```python
from build123d import *
from build123d.topology import SkipClean

# Parameters (mm, degrees)
SKETCH2_R               = 22.5
BOSS_EXTRUDE1_DEPTH     = 8
SKETCH3_R               = 5
BOSS_EXTRUDE2_DEPTH     = 70
SKETCH4_R               = 12
BOSS_EXTRUDE3_DEPTH     = 28
FILLET1_R               = 6
CUT_EXTRUDE1_DEPTH      = 85.240726493
CUT_EXTRUDE1_DEPTH_BACK = 85.240726493
SKETCH5_W               = 15
SKETCH5_H               = 20
SKETCH6_R               = 4
CUT_EXTRUDE2_DEPTH      = 28
SKETCH7_R               = 9
SKETCH7_R_2             = 4
BOSS_EXTRUDE5_DEPTH     = 12.5
FILLET3_R               = 1


with BuildPart() as part:
    # Sketch2 → Boss-Extrude1 (new body)
    with BuildSketch(Plane(origin=(0, 0, 0), x_dir=(1, 0, 0), z_dir=(0, 1, 0))):
        with Locations(Location((0, 0, 0), (0, 0, 270))):
            Circle(SKETCH2_R)
    extrude(amount=BOSS_EXTRUDE1_DEPTH)

    # Sketch3 → Boss-Extrude2 (add)
    with BuildSketch(Plane(origin=(0, 8, 0), x_dir=(1, 0, 0), z_dir=(0, 1, 0))):
        with Locations(Location((0, 0, 0), (0, 0, 270))):
            Circle(SKETCH3_R)
    extrude(amount=BOSS_EXTRUDE2_DEPTH)

    # Sketch4 → Boss-Extrude3 (add)
    with BuildSketch(Plane.XZ):
        with Locations(Location((0, 0, 0), (0, 0, 270))):
            Circle(SKETCH4_R)
    extrude(amount=BOSS_EXTRUDE3_DEPTH)

    # Fillet1
    fillet1_edges = [part.edges().sort_by_distance(p)[0] for p in [
        (0, -28, 12),
    ]]
    fillet(fillet1_edges, radius=FILLET1_R)

    # Sketch5 → Cut-Extrude1 (cut, two sides: drawn at the far end of the back side and taken through both)
    with BuildSketch(Plane(origin=(0, 0, 0), x_dir=(0, 0, -1), z_dir=(1, 0, 0)).offset(-CUT_EXTRUDE1_DEPTH_BACK)):
        with Locations((15, -18)):
            Rectangle(SKETCH5_W, SKETCH5_H)
        with Locations((-15, -18)):
            Rectangle(SKETCH5_W, SKETCH5_H)
    extrude(amount=CUT_EXTRUDE1_DEPTH + CUT_EXTRUDE1_DEPTH_BACK, mode=Mode.SUBTRACT)

    # Sketch6 → Cut-Extrude2 (cut)
    with BuildSketch(Plane(origin=(0, 0, -7.5), x_dir=(-1, 0, 0), z_dir=(0, 0, -1))):
        with Locations(Location((0, -18, 0), (0, 0, 90))):
            Circle(SKETCH6_R)
    extrude(amount=-CUT_EXTRUDE2_DEPTH, mode=Mode.SUBTRACT)

    # Sketch7 → Boss-Extrude5 (add, symmetric)
    with SkipClean():  # the faces are left unmerged after this step: merging them gives an invalid solid
        with BuildSketch(Plane.XY):
            with Locations(Location((0, -18, 0), (0, 0, 180))):
                Circle(SKETCH7_R)
            with Locations((0, -18)):
                Circle(SKETCH7_R_2, mode=Mode.SUBTRACT)
        extrude(amount=BOSS_EXTRUDE5_DEPTH, both=True)
    add(part.part.scale(1), mode=Mode.REPLACE)  # the faces are merged on a copy

    # Fillet3
    fillet3_edges = [part.edges().sort_by_distance(p)[0] for p in [
        (0, 0, -22.5),
    ]]
    fillet(fillet3_edges, radius=FILLET3_R)


solid = part.part
```
Read the model definition and answer for the solid it produces. Units are mm, in the model's axes. A direction names the side the tool comes from. Coordinates: 2 decimals unless noted, no trailing zeros. Loops run counter-clockwise (first coordinate to the right, second up) from the corner with the lowest first, then second, coordinate; pieces in that order, holes last.
(1) The mould has two halves that part along Y. Classify faces 4 (the face through (0, -8, -9)), 5 (the face through (1.172, -26.923, 10.035)), 6 (the face through (0, -28, 0)), 7 (the face through (-8.618, 4.451, 20.784)): released by +Y, released by -Y, zero draft, split by the parting line, or undercut.
Solution:
face 4: undercut
face 5: undercut
face 6: released by -Y
face 7: zero draft
(2) A tool of negligible diameter and unlimited length cuts with its end or side. For faces 1 (the face through (-2, -14, 12.5)), 2 (the face through (2, -9, -7.5)), 3 (the face through (-4.88, 42.51, -1.08)), from which of +Z, -Z, +X, -X, +Y, -Y can it reach the whole face along a straight path? Write none if from no direction.
Solution:
face 1: +Z, +X, -X, -Y
face 2: -Z
face 3: +Y
(3) The part is cut by section A-A (y = 15.5). Determine the outline of the cut face in (x, z), and give its area (3 significant figures).
Solution:
outline: circle Ø10 at (0, 0)
area: 78.5 mm2
(4) Consider line 1 along X through (y, z) = (-18, -10); line 2 along Y through (x, z) = (0, 4); line 3 along X through (y, z) = (-18, 5). Determine where each line is inside the solid, lowest interval first.
Solution:
line 1: x = -9 to -4, 4 to 9
line 2: y = -28 to -22, -14 to 78
line 3: x = -10.91 to -4, 4 to 10.91
(5) Flat-ended cylindrical pins translate along their axes: pin 1 Ø9 at (x, y) = (0, -18) entering from +Z; pin 2 Ø4 at (x, y) = (16.5, 7.5) entering from +Z; pin 3 Ø3 at (x, y) = (-2, 14.5) entering from +Z; pin 4 Ø5 at (x, y) = (0, -18) entering from -Z. Find the tip coordinate at first contact, or state that the pin passes through.
Solution:
pin 1: stops at z = 12.5
pin 2: stops at z = 17.2
pin 3: stops at z = 4.97
pin 4: passes through
